```python
from build123d import *

# Parameters (mm, degrees)
F1_DEPTH    = 56
F2_T1_DEPTH = 363.4104337306
F3_DEPTH    = 56
F6_DEPTH    = 6
F5_W        = 259.5228254795
F5_H        = 121.416632086
F7_DEPTH    = 25
F8_DEPTH    = 52


# Not quite as in the source:
# - a fillet or chamfer that OpenCascade refuses, or shapes differently, is made with other operations: its cross-section is extruded or revolved along the edge and cut away or added


with BuildPart() as f1:
    # F0 (on Top) → F1 (new body)
    with BuildSketch(Plane.XY):
        Polygon((80, -24), (-80, -24), (-58.2867488807, 13.6084541361), (-65.214952111, 13.6084541361), (-73.0717967697, 0), (-90.3923048454, -30), (90.3923048454, -30), (73.0717967697, 0), (65.214952111, 13.6084541361), (58.2867488807, 13.6084541361), align=None)
        Polygon((-90.3923048454, -30), (-73.0717967697, 0), (-90.3923048454, 0), align=None)
        Polygon((90.3923048454, 0), (73.0717967697, 0), (90.3923048454, -30), align=None)
        Polygon((-73.0717967697, 0), (-65.214952111, 13.6084541361), (-90.3923048454, 13.6084541361), (-90.3923048454, 0), align=None)
        Polygon((90.3923048454, 13.6084541361), (65.214952111, 13.6084541361), (73.0717967697, 0), (90.3923048454, 0), align=None)
    extrude(amount=F1_DEPTH)

    # F2: chamfer of 25 x 35.3610857633 on 1 edges, made by hand

    # F2_s2 → F2_t1 (cut)
    with BuildSketch(Plane.YZ.offset(-181.7052168653)):
        Polygon((-30, 31), (5.3610857633, 56), (-30, 56), align=None)
    extrude(amount=F2_T1_DEPTH, mode=Mode.SUBTRACT)

    # F0 (on Top) → F3 (join)
    with BuildSketch(Plane.XY):
        Polygon((-58.2867488807, 13.6084541361), (-80, -24), (80, -24), (58.2867488807, 13.6084541361), align=None)
    extrude(amount=F3_DEPTH)

    # F0 (on Top) → F6 (join)
    with BuildSketch(Plane.XY):
        Polygon((-58.2867488807, 13.6084541361), (-80, -24), (80, -24), (58.2867488807, 13.6084541361), align=None)
        Polygon((80, -24), (-80, -24), (-58.2867488807, 13.6084541361), (-65.214952111, 13.6084541361), (-73.0717967697, 0), (-90.3923048454, -30), (90.3923048454, -30), (73.0717967697, 0), (65.214952111, 13.6084541361), (58.2867488807, 13.6084541361), align=None)
        Polygon((-90.3923048454, -30), (-73.0717967697, 0), (-90.3923048454, 0), align=None)
        Polygon((-73.0717967697, 0), (-65.214952111, 13.6084541361), (-90.3923048454, 13.6084541361), (-90.3923048454, 0), align=None)
        Polygon((90.3923048454, 13.6084541361), (65.214952111, 13.6084541361), (73.0717967697, 0), (90.3923048454, 0), align=None)
        Polygon((90.3923048454, 0), (73.0717967697, 0), (90.3923048454, -30), align=None)
    extrude(amount=-F6_DEPTH)

    # F5 (on offset) → F7 (cut)
    with BuildSketch(Plane(origin=(0, -24.6105813664, 34.8102751353), x_dir=(1, 0, 0), z_dir=(0, -0.5772877121, 0.8165408119))):
        with Locations((5.841344595, -0.7894355804)):
            Rectangle(F5_W, F5_H)
    extrude(amount=F7_DEPTH, mode=Mode.SUBTRACT)

    # F0 (on Top) → F8 (cut)
    with BuildSketch(Plane.XY):
        Polygon((-58.2867488807, 13.6084541361), (-80, -24), (80, -24), (58.2867488807, 13.6084541361), align=None)
    extrude(amount=F8_DEPTH, mode=Mode.SUBTRACT)


solid = f1.part
```
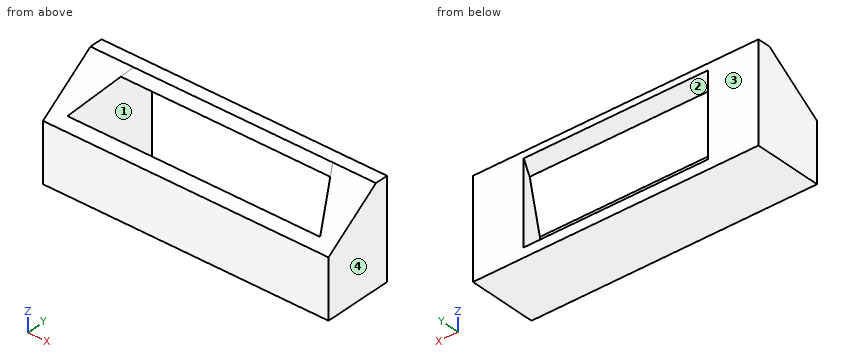
Geometry check sheet. Reference: the model listing, model coordinates, mm. Face numbers are marked on the shaded views. Round coordinates to 2 decimals unless told otherwise and drop trailing zeros. Order: outer loops, then holes, each group sorted by start corner. A loop starts at its lowest first (then second) coordinate and runs counter-clockwise, first axis right, second up. Notation, with made-up numbers: (75, -34) - (81, -34) arc R16 cw to (81, -18) - close; hole circle Ø11 at (51.5, 44.5). An arc over 180 degrees is marked (long way). Use a Markdown table: item, result. Add a question column.
(1) Release check for a two-part mould opening along X. For the marked faces 1, 2, 3 and 4 record: pulls with the +X half, pulls with the -X half, needs draft (parallel to the pull), parting line crosses it, or undercut.
(2) Sectioned sample at C-C, the plane y = 9. Enter the section's corners in (x, z), and give its area (3 significant figures).
(3) Sectioned sample at B-B, the plane z = 44. Enter the section's corners in (x, y), and give its area (3 significant figures).
(4) Depth check by flat-ended pin: pin 1 (8 mm diameter, centred on x = 41.5, z = 17.5, fed in from +Y); pin 2 (11.5 mm diameter, centred on x = -13.5, y = -8, fed in from +Z); pin 3 (4 mm diameter, centred on x = -32.5, y = -25, fed in from +Z). Enter the tip coordinate at first touch or a pass-through.
(5) Material ranges on line 1 along Z through (x, y) = (46, 7); line 2 along Y through (x, z) = (-56.5, 26.5); line 3 along Z through (x, y) = (44.5, -18.5), recorded low to high. Write a range as [from, to].
(6) Sectioned sample at A-A, the plane x = 13.5. Enter the section's corners in (y, z).
(7) Sectioned sample at D-D, the plane z = 2. Enter the section's corners in (x, y).
Answers below:
| question | item | result |
|---|---|---|
| 1 | face 1 | undercut |
| 1 | face 2 | undercut |
| 1 | face 3 | needs draft |
| 1 | face 4 | pulls with the +X half |
| 2 | outline | (-90.39, -6) - (90.39, -6) - (90.39, 56) - (-90.39, 56) - close; hole (-60.95, 0) - (60.95, 0) - (60.95, 52) - (-60.95, 52) - close |
| 2 | area | 4,870 mm² |
| 3 | outline | (-90.39, -11.61) - (-72.85, -11.61) - (-58.29, 13.61) - (-90.39, 13.61) - close; (58.29, 13.61) - (72.85, -11.61) - (90.39, -11.61) - (90.39, 13.61) - close |
| 3 | area | 1,250 mm² |
| 4 | pin 1 | y = -24 |
| 4 | pin 2 | z = 0 |
| 4 | pin 3 | z = 35.24 |
| 5 | line 1 | [-6, 0], [52, 56] |
| 5 | line 2 | [-30, -24] |
| 5 | line 3 | [-6, 0] |
| 6 | outline | (-30, -6) - (13.61, -6) - (13.61, 0) - (-24, 0) - (-24, 35.24) - (-30, 31) - close; (-0.3, 52) - (13.61, 52) - (13.61, 56) - (5.36, 56) - close |
| 7 | outline | (-90.39, -30) - (90.39, -30) - (90.39, 13.61) - (58.29, 13.61) - (80, -24) - (-80, -24) - (-58.29, 13.61) - (-90.39, 13.61) - close |
